```python
from build123d import *

# Parameters (mm, degrees)
SKETCH1_R           = 7.5
SKETCH1_R_2         = 4
BOSS_EXTRUDE1_DEPTH = 24
SKETCH2_R           = 6.5
SKETCH2_R_2         = 4.5
CUT_EXTRUDE1_DEPTH  = 0.4
SKETCH3_W           = 1.1
SKETCH3_H           = 0.6
CHAMFER1_SIZE       = 0.5
CHAMFER2_SIZE       = 0.2


with BuildPart() as part:
    # Sketch1 → Boss-Extrude1 (new body)
    with BuildSketch(Plane.XY):
        Circle(SKETCH1_R)
        Circle(SKETCH1_R_2, mode=Mode.SUBTRACT)
    extrude(amount=BOSS_EXTRUDE1_DEPTH)

    # Sketch2 → Cut-Extrude1 (cut)
    with BuildSketch(Plane.XY.offset(24)):
        Circle(SKETCH2_R)
        Circle(SKETCH2_R_2, mode=Mode.SUBTRACT)
    cut_extrude1 = extrude(amount=-CUT_EXTRUDE1_DEPTH, mode=Mode.SUBTRACT)

    # Mirror1: Cut-Extrude1 across plane
    add(cut_extrude1.mirror(Plane.XY.offset(12)), mode=Mode.SUBTRACT)

    # Sketch3 → Cut-Revolve1 (revolve, cut)
    with BuildSketch(Plane(origin=(0, 0, 0), x_dir=(0, 0, -1), z_dir=(1, 0, 0)), mode=Mode.PRIVATE) as cut_revolve1_sk:
        with Locations((-20.2, 7.2)):
            Rectangle(SKETCH3_W, SKETCH3_H)
        with Locations((-3.8, 7.2)):
            Rectangle(SKETCH3_W, SKETCH3_H)
    revolve(cut_revolve1_sk.sketch.rotate(Axis((0, 0, 24), (0, 0, -1)), 90), axis=Axis((0, 0, 24), (0, 0, -1)), mode=Mode.SUBTRACT)

    # Chamfer1
    chamfer1_edges = [part.edges().sort_by_distance(p)[0] for p in [
        (-7.5, 0, 0),
        (-7.5, 0, 24),
    ]]
    chamfer(chamfer1_edges, length=CHAMFER1_SIZE)

    # Chamfer2
    chamfer2_edges = [part.edges().sort_by_distance(p)[0] for p in [
        (-7.5, 0, 20.75),
        (-7.5, 0, 19.65),
        (-7.5, 0, 4.35),
        (-7.5, 0, 3.25),
    ]]
    chamfer(chamfer2_edges, length=CHAMFER2_SIZE)


solid = part.part
```
Work out the finished part from the listing and answer in its coordinate system (mm). A direction names the side the tool comes from. Give positions to 0.01 mm unless a question says otherwise; leave off trailing zeros. Write each loop counter-clockwise with the first axis right and the second up, starting at its lowest first coordinate (ties: lowest second). Pieces come first, ordered by that corner, then holes. Notation, with made-up numbers: (-9, -39.5) -> (25, -39.5) arc R11 ccw to (25, -28.5) -> close; hole circle Ø4 at (19, -36). An arc over 180 degrees is marked (long way). Write item = value, one per line.
Q1. Consider line 1 along Z through (x, y) = (-6.5, 3.25); line 2 along Y through (x, z) = (-2.5, 11); line 3 along X through (y, z) = (-3, 7.5). Determine where each line is inside the solid, lowest interval first.
Computed values:
line_1 = 0.27 to 3.25, 4.35 to 19.65, 20.75 to 23.73
line_2 = -7.07 to -3.12, 3.12 to 7.07
line_3 = -6.87 to -2.65, 2.65 to 6.87
Q2. Section B-B on z = 3.75 is taken. Determine the outline of the cut face in (x, y).
Computed values:
outline = circle Ø13.8 at (0, 0); hole circle Ø8 at (0, 0)
Q3. Flat-ended cylindrical pins translate along their axes: pin 1 Ø4 at (x, z) = (-5.5, 2.5) entering from -Y; pin 2 Ø1 at (y, z) = (-4, 8) entering from +X; pin 3 Ø4 at (x, z) = (6, 19.5) entering from +Y. Find the tip coordinate at first contact, or state that the pin passes through.
Computed values:
pin_1 = -6.63
pin_2 = 6.63
pin_3 = 6.34
Q4. For a pull along Y with two mould halves and no side action, classify faces 4 (the cylindrical face through (-5.158, -3.955, 0.197)), 5 (the cylindrical face through (-5.09, -4.66, 3.79)), 6 (the flat face through (-3, -3, 0)), 7 (the cylindrical face through (-0.59, 4.46, 23.8)) as pulls with the +Y half, pulls with the -Y half, needs draft (parallel to the pull), parting line crosses it, or undercut.
Computed values:
face_4 = undercut
face_5 = parting line crosses it
face_6 = needs draft
face_7 = undercut
Q5. A tool of negligible diameter and unlimited length cuts with its end or side. For faces 1 (the cylindrical face through (-5.09, -4.66, 20.19)), 2 (the cylindrical face through (-5.158, -3.955, 23.803)), 3 (the flat face through (-4.42, 1.54, 0.4)), from which of +Z, -Z, +X, -X, +Y, -Y can it reach the whole face along a straight path? Write none if from no direction.
Computed values:
face_1 = none
face_2 = +Z
face_3 = -Z
Q6. Section A-A on z = 12.5 is taken. Determine the outline of the cut face in (x, y), and give its area (3 significant figures).
Computed values:
outline = circle Ø15 at (0, 0); hole circle Ø8 at (0, 0)
area = 126 mm^2
